Verification items for the finished model (mm, model axes). Face numbers are marked on the shaded views. A direction names the side the tool comes from. Round coordinates to 2 decimals unless told otherwise and drop trailing zeros. Write each loop counter-clockwise with the first axis right and the second up, starting at its lowest first coordinate (ties: lowest second). Pieces come first, ordered by that corner, then holes. Notation, with made-up numbers: (13, -5) - (59, -5) arc R23 cw to (59, 13) - close; hole circle Ø4 at (-7, 34). An arc over 180 degrees is marked (long way). Answer as a JSON object with one key per item and string values. Group by question number.
1) Section check B-B (x = 0). Enter the section's corners in (y, z).
2) Section check A-A (z = 4.2). Enter the section's corners in (x, y).
3) Section check C-C (z = 2.45). Enter the section's corners in (x, y).
4) Mould release check, pull along Z, two halves, no side actions. Record for the marked faces 6, 7 and 8: +Z half, -Z half, draft (parallel to the pull), parting line (faces both ways), or undercut.
5) Set-up check for the marked faces 1, 2, 3, 4 and 5: record each of +Z, -Z, +X, -X, +Y, -Y from which the full face is reachable in a straight line by a thin tool's end or side.
6) Thickness scan on line 1 (Z direction, x = 0.15, y = -0.85); line 2 (X direction, y = 1.65, z = 3.55); line 3 (Z direction, x = -2.3, y = -0.1). Record the ranges inside material, lowest first.
7) Go/stop test with flat-tipped pins: pin 1 Ø2.5 at (x, y) = (0, 0.5) entering from +Z; pin 2 Ø0.5 at (x, z) = (-2.5, 0.5) entering from +Y; pin 3 Ø3 at (x, y) = (-1, -1) entering from -Z; pin 4 Ø0.8 at (y, z) = (0, 4) entering from -X. Record where each tip stops, or that it passes through.
```python
from build123d import *

# Parameters (mm, degrees)
SKETCH_W     = 6
SKETCH_H     = 6
PAD_DEPTH    = 1
POCKET_DEPTH = 1
SKETCH002_R  = 2.4
PAD001_DEPTH = 2.5
FILLET_R     = 0.5
SKETCH003_W  = 5
SKETCH003_H  = 6
PAD002_DEPTH = 1
CHAMFER_SIZE = 1
FILLET001_R  = 0.25
PAD003_DEPTH = 0.1
SKETCH005_W  = 2.980372
SKETCH005_H  = 0.513015
PAD004_DEPTH = 0.05


with BuildPart() as part:
    # Sketch → Pad (new body)
    with BuildSketch(Plane.XY):
        Rectangle(SKETCH_W, SKETCH_H)
    extrude(amount=PAD_DEPTH)

    # Sketch001 (on Face6 of Pad) → Pocket (cut)
    with BuildSketch(Plane.XY.offset(1)):
        Polygon((-3, 3), (-3, 2.465282), (-2.429642, 2.465282), (-2.036143, 3), align=None)
        Polygon((3, 3), (3, 2.465282), (2.429642, 2.465282), (2.036143, 3), align=None)
        Polygon((-3, -3), (-3, -2.465282), (-2.429642, -2.465282), (-2.036143, -3), align=None)
        Polygon((3, -3), (3, -2.465282), (2.429642, -2.465282), (2.036143, -3), align=None)
    extrude(amount=-POCKET_DEPTH, mode=Mode.SUBTRACT)

    # Sketch002 (on Face4 of Pocket) → Pad001 (join)
    with BuildSketch(Plane.XY.offset(1)):
        Circle(SKETCH002_R)
    extrude(amount=PAD001_DEPTH)

    # Fillet
    fillet_edges = [part.edges().sort_by_distance(p)[0] for p in [
        (-2.4, 0, 1),
    ]]
    fillet(fillet_edges, radius=FILLET_R)

    # Sketch003 (on Face17 of Fillet) → Pad002 (join)
    with BuildSketch(Plane.XY.offset(3.5)):
        Rectangle(SKETCH003_W, SKETCH003_H)
    extrude(amount=PAD002_DEPTH)

    # Chamfer
    chamfer_edges = [part.edges().sort_by_distance(p)[0] for p in [
        (-2.5, -3, 4),
        (2.5, -3, 4),
        (-2.5, 3, 4),
        (2.5, 3, 4),
    ]]
    chamfer(chamfer_edges, length=CHAMFER_SIZE)

    # Fillet001
    fillet001_edges = [part.edges().sort_by_distance(p)[0] for p in [
        (-2.4, 0, 3.5),
    ]]
    fillet(fillet001_edges, radius=FILLET001_R)

    # Sketch004 (on Face32 of Fillet001) → Pad003 (join)
    with BuildSketch(Plane(origin=(0, 0, 0), x_dir=(1, 0, 0), z_dir=(0, 0, -1))):
        Polygon((-2.914238, 1.375165), (-2.921686, -1.414024), (-2.649441, -1.406666), (-2.656799, -2.39999), (-2.369838, -2.407348), (-2.178532, -2.701667), (-1.928361, -2.694309), (-1.928272, 2.80261), (-2.119579, 2.80261), (-2.421255, 2.397922), (-2.6935, 2.397922), (-2.6935, 1.367807), align=None)
    pad003 = extrude(amount=PAD003_DEPTH)

    # Mirrored: Pad003 across YZ
    add(pad003.mirror(Plane.YZ))

    # Sketch005 (on Face10 of Mirrored) → Pad004 (join)
    with BuildSketch(Plane.XY.offset(4.5)):
        with Locations((0.026899, -1.174543)):
            Rectangle(SKETCH005_W, SKETCH005_H)
    extrude(amount=PAD004_DEPTH)


solid = part.part
```
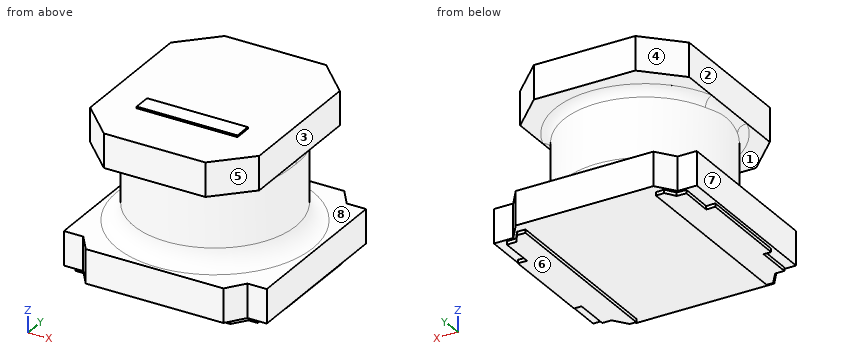
Returned:
{
 "1": {"outline": "(-3, 0) - (3, 0) - (3, 1) - (2.9, 1) arc R0.5 cw to (2.4, 1.5) - (2.4, 3.25) arc R0.25 cw to (2.65, 3.5) - (3, 3.5) - (3, 4.5) - (-0.92, 4.5) - (-0.92, 4.55) - (-1.43, 4.55) - (-1.43, 4.5) - (-3, 4.5) - (-3, 3.5) - (-2.65, 3.5) arc R0.25 cw to (-2.4, 3.25) - (-2.4, 1.5) arc R0.5 cw to (-2.9, 1) - (-3, 1) - close"},
 "2": {"outline": "(-2.5, -2) - (-1.5, -3) - (1.5, -3) - (2.5, -2) - (2.5, 2) - (1.5, 3) - (-1.5, 3) - (-2.5, 2) - close"},
 "3": {"outline": "circle Ø4.8 at (0, 0)"},
 "4": {"face 6": "-Z half", "face 7": "draft", "face 8": "undercut"},
 "5": {"face 1": "-Y", "face 2": "+Z, -X, +Y, -Y", "face 3": "+Z, +X, +Y, -Y", "face 4": "+Z, -X, +Y", "face 5": "+Z, +X, -Y"},
 "6": {"line 1": "0 to 4.5", "line 2": "-2.5 to 2.5", "line 3": "-0.1 to 4.5"},
 "7": {"pin 1": "z = 4.5", "pin 2": "y = 2.71", "pin 3": "z = -0.1", "pin 4": "x = -2.5"}
}
